For this review, take the finished solid that the model builds, in its own axes (mm). Face numbers are marked on the shaded views. A direction names the side the tool comes from. Give positions to 0.01 mm unless a question says otherwise; leave off trailing zeros. Write each loop counter-clockwise with the first axis right and the second up, starting at its lowest first coordinate (ties: lowest second). Pieces come first, ordered by that corner, then holes.
Q1. Mouldability with a two-part tool opening along Y and no side actions: class the marked faces 1, 2, 3 and 4 as released by +Y, released by -Y, zero draft, split by the parting line, or undercut.
Q2. Insertion check: P1, Ø1.8, axis at y = 15.5, z = 11.5, coming from the +X side. The pin has a flat end and moves straight along its axis. Give the tip position at first contact, or say it passes through.
Q3. We need section D-D (z = 17). Write out the cut boundary in (x, y), then the cut area to 3 significant figures.
Q4. We need section B-B (x = -3.25). Write out the cut boundary in (y, z), then the cut area to 3 significant figures.
Q5. For line 1 (Y direction, x = -17.75, z = 14); line 2 (Z direction, x = -2.75, y = 6.75); line 3 (Y direction, x = -12.25, z = 17.25), list the stretches that pass through material, from the lowest coordinate up.
Q6. Machinability: for the marked faces 5, 6 and 7, which of the approach directions +Z, -Z, +X, -X, +Y, -Y give a long, thin tool a straight path to every point of the face, cutting with its end or side? Answer none if there is none.
Q7. We need section C-C (z = 12). Write out the cut boundary in (x, y), then the cut area to 4 significant figures.
Q8. We need section A-A (y = 5.75). Write out the cut boundary in (x, z).
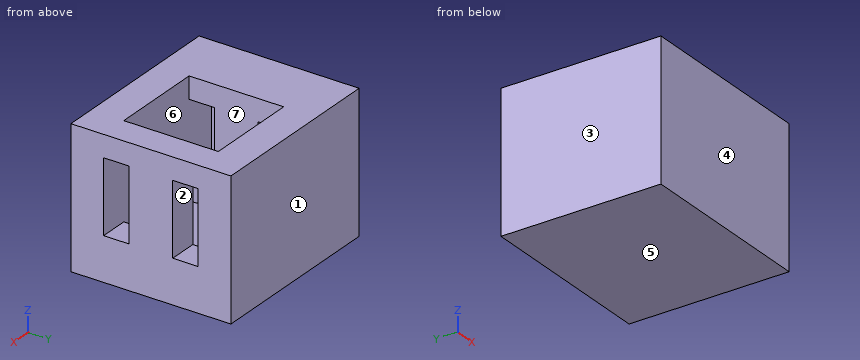
```python
from build123d import *

# Parameters (mm, degrees)
F0_W     = 4.5
F0_H     = 3
F1_DEPTH = 16
F2_DEPTH = 6
F3_DEPTH = 3
F0_W_2   = 4
F4_DEPTH = 16
F5_W     = 4.5
F5_H     = 3.5
F5_W_2   = 4
F5_H_2   = 13
F6_DEPTH = 3


with BuildPart() as f1:
    # F0 (on Top) → F1 (new body)
    with BuildSketch(Plane.XY):
        Polygon((-25.5, 22), (-25.5, 11), (-21.5, 11), (-17, 11), (-17, 14), (-21.5, 14), (-21.5, 14.5), (-21.5, 17.5), (-17, 17.5), (-4, 17.5), (0, 17.5), (0, 22), align=None)
        Polygon((-25.5, 0), (0, 0), (0, 4.5), (-4, 4.5), (-17, 4.5), (-21.5, 4.5), (-21.5, 7.5), (-21.5, 8), (-21.5, 11), (-25.5, 11), align=None)
        with Locations((-19.25, 9.5)):
            Rectangle(F0_W, F0_H)
    extrude(amount=F1_DEPTH)

    # F0 (on Top) → F2 (join)
    with BuildSketch(Plane.XY):
        Polygon((-21.5, 4.5), (-17, 4.5), (-17, 5), (-17, 7.5), (-17, 8), (-21.5, 8), (-21.5, 7.5), align=None)
        Polygon((-21.5, 14), (-17, 14), (-17, 14.5), (-17, 17), (-17, 17.5), (-21.5, 17.5), (-21.5, 14.5), align=None)
        Polygon((0, 17), (0, 17.5), (-4, 17.5), (-4, 17), (-4, 14), (0, 14), (0, 14.5), align=None)
        Polygon((-4, 4.5), (0, 4.5), (0, 5), (0, 7.5), (0, 8), (-4, 8), (-4, 7.5), (-4, 5), align=None)
    extrude(amount=F2_DEPTH)

    # F0 (on Top) → F3 (join)
    with BuildSketch(Plane.XY):
        Polygon((-17, 14), (-17, 11), (-16.5, 11), (-4, 11), (-4, 14), (-4, 17), (-4, 17.5), (-17, 17.5), (-17, 17), (-17, 14.5), align=None)
        Polygon((-17, 4.5), (-4, 4.5), (-4, 5), (-4, 7.5), (-4, 8), (-4, 11), (-16.5, 11), (-17, 11), (-17, 8), (-17, 7.5), (-17, 5), align=None)
    extrude(amount=F3_DEPTH)

    # F0 (on Top) → F4 (join)
    with BuildSketch(Plane.XY):
        with Locations((-2, 9.5)):
            Rectangle(F0_W_2, F0_H)
        with Locations((-2, 12.5)):
            Rectangle(F0_W_2, F0_H)
    extrude(amount=F4_DEPTH)

    # F5 (on face) → F6 (join)
    with BuildSketch(Plane.XY.offset(16)):
        with Locations((-19.25, 6.25)):
            Rectangle(F5_W, F5_H)
        with Locations((-19.25, 15.75)):
            Rectangle(F5_W, F5_H)
        with Locations((-2, 11)):
            Rectangle(F5_W_2, F5_H_2)
        Polygon((0, 4.5), (-4, 4.5), (-17, 4.5), (-21.5, 4.5), (-21.5, 8), (-17, 8), (-17, 14), (-21.5, 14), (-21.5, 17.5), (-17, 17.5), (-4, 17.5), (0, 17.5), (0, 22), (-25.5, 22), (-25.5, 0), (0, 0), align=None)
    extrude(amount=F6_DEPTH)


solid = f1.part
```
Computed:
1. face 1: released by +Y
1. face 2: undercut
1. face 3: zero draft
1. face 4: released by -Y
2. P1: stops at x = -21.5
3. outline: (-25.5, 0) - (0, 0) - (0, 22) - (-25.5, 22) - close; hole (-17, 4.5) - (-4, 4.5) - (-4, 17.5) - (-17, 17.5) - close
3. area: 392 mm2
4. outline: (0, 0) - (22, 0) - (22, 19) - (0, 19) - close; hole (4.5, 6) - (8, 6) - (8, 16) - (4.5, 16) - close; hole (14, 6) - (17.5, 6) - (17.5, 16) - (14, 16) - close
4. area: 348 mm2
5. line 1: y = 0 to 4.5, 8 to 14, 17.5 to 22
5. line 2: z = 0 to 6, 16 to 19
5. line 3: y = 0 to 4.5, 17.5 to 22
6. face 5: -Z, +X, -X, +Y, -Y
6. face 6: none
6. face 7: +Z
7. outline: (-25.5, 0) - (0, 0) - (0, 4.5) - (-21.5, 4.5) - (-21.5, 8) - (-17, 8) - (-17, 14) - (-21.5, 14) - (-21.5, 17.5) - (0, 17.5) - (0, 22) - (-25.5, 22) - close; (-4, 8) - (0, 8) - (0, 14) - (-4, 14) - close
7. area: 332.5 mm2
8. outline: (-25.5, 0) - (0, 0) - (0, 6) - (-4, 6) - (-4, 3) - (-17, 3) - (-17, 6) - (-21.5, 6) - (-21.5, 16) - (-17, 16) - (-17, 19) - (-25.5, 19) - close; (-4, 16) - (0, 16) - (0, 19) - (-4, 19) - close
